Could you check a few things on this model? Use its own coordinates, in mm. Face numbers are marked on the shaded views. Round coordinates to 2 decimals unless told otherwise and drop trailing zeros. Loops run counter-clockwise (first coordinate to the right, second up) from the corner with the lowest first, then second, coordinate; pieces in that order, holes last. Notation, with made-up numbers: M -37.5,52 L -23.5,52 A37 ccw -23.5,88 Z; hole C 68,29.5 d10. An arc over 180 degrees is marked long. Answer in a Markdown table with one row per item.
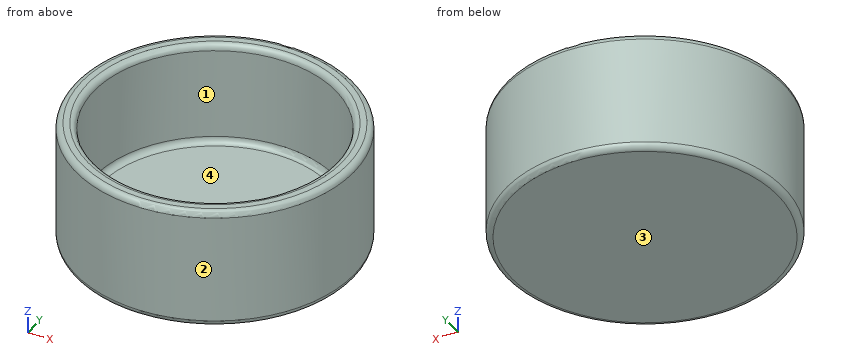
```python
from build123d import *

# Parameters (mm, degrees)
F0_R     = 23
F0_R_2   = 20
F1_DEPTH = 20
F2_R     = 23
F3_DEPTH = 3
F4_R     = 1


with BuildPart() as f1:
    # F0 (on Top) → F1 (new body)
    with BuildSketch(Plane.XY):
        Circle(F0_R)
        Circle(F0_R_2, mode=Mode.SUBTRACT)
    extrude(amount=F1_DEPTH)

    # F2 (on Top) → F3 (join)
    with BuildSketch(Plane.XY):
        Circle(F2_R)
    extrude(amount=F3_DEPTH)

    # F4
    f4_edges = [f1.edges().sort_by_distance(p)[0] for p in [
        (-20, 0, 3),
        (-20, 0, 20),
        (-23, 0, 20),
        (-23, 0, 0),
        (23, 0, 10),
    ]]
    fillet(f4_edges, radius=F4_R)


solid = f1.part
```
1) I want a section at B-B, the plane x = 0. Please give me the cut outline in (y, z), plus the area to 3 significant figures.
Computed:
| item | result |
|---|---|
| outline | M -23,1 A1 ccw -22,0 L 22,0 A1 ccw 23,1 L 23,19 A1 ccw 22,20 L 21,20 A1 ccw 20,19 L 20,4 A1 cw 19,3 L -19,3 A1 cw -20,4 L -20,19 A1 ccw -21,20 L -22,20 A1 ccw -23,19 Z |
| area | 239 mm² |
2) I need wall thicknesses on line 1 (Y direction, x = 0, z = 9.5); line 2 (Z direction, x = -7.5, y = 1); line 3 (Y direction, x = 16, z = 8.75). Which ranges of each line are inside material? Lowest first, please.
Computed:
| item | result |
|---|---|
| line 1 | y = -23 to -20, 20 to 23 |
| line 2 | z = 0 to 3 |
| line 3 | y = -16.52 to -12, 12 to 16.52 |
3) If we mould it in two halves opening along X, with no side actions, what happens to the marked faces 1, 2, 3 and 4? For each: released by +X, released by -X, zero draft, split by the parting line, or undercut.
Computed:
| item | result |
|---|---|
| face 1 | undercut |
| face 2 | split by the parting line |
| face 3 | zero draft |
| face 4 | undercut |
4) I want a section at A-A, the plane z = 13. Please give me the cut outline in (x, y), plus the area to 3 significant figures.
Computed:
| item | result |
|---|---|
| outline | C 0,0 d46; hole C 0,0 d40 |
| area | 405 mm² |
5) Will these pins go through, and if not, where does the flat tip stop? P1, Ø8, axis at x = -9.5, z = 7.5, coming from the +Y side; P2, Ø3, axis at x = -16, z = 17, coming from the -Y side; P3, Ø3, axis at x = -18, z = 3.5, coming from the +Y side; P4, Ø5, axis at x = -15, y = -14, coming from the +Z side.
Computed:
| item | result |
|---|---|
| P1 | stops at y = 22.33 |
| P2 | stops at y = -17.85 |
| P3 | stops at y = 16.02 |
| P4 | stops at z = 20 |
